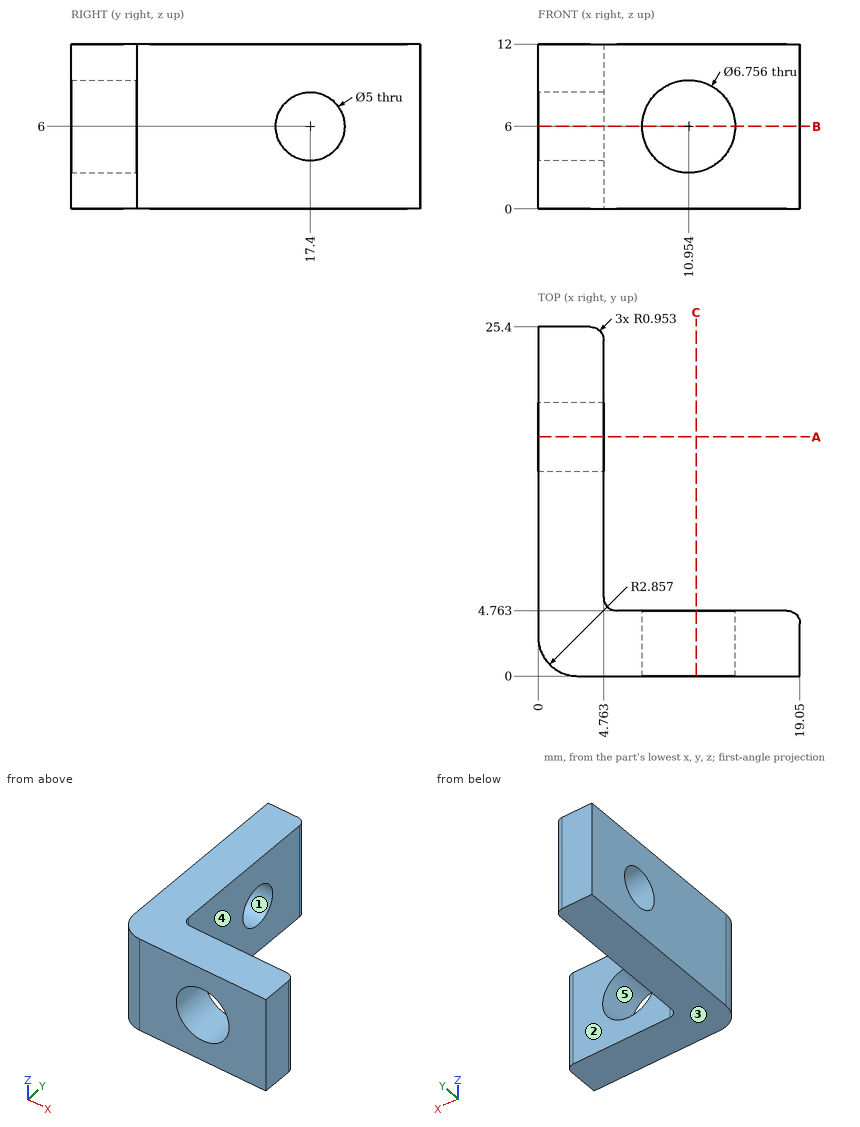
Answer from the drawing. Dimensions are ordinates in mm from the lowest x, y and z of the part. A direction names the side the tool comes from. Round coordinates to 2 decimals unless told otherwise and drop trailing zeros. Write each loop counter-clockwise with the first axis right and the second up, starting at its lowest first coordinate (ties: lowest second). Pieces come first, ordered by that corner, then holes. Notation, with made-up numbers: M -19.5,77 L 36.5,77 A14 cw 36.5,98 Z; hole C 85.5,65 d3. An arc over 180 degrees is marked long. Write each question's results on one line, items separated by ' | '. Start each with the question number.
Item 1: The mould has two halves that part along Z. Classify the marked faces 1, 2 and 3: +Z half, -Z half, draft (parallel to the pull), parting line (faces both ways), or undercut.
Item 2: Find section C-C on x = 11.5. Write down the section's boundary in (y, z).
Item 3: Given pin 1 Ø6 at (x, z) = (10.5, 8) entering from +Y; pin 2 Ø5 at (x, z) = (5, 7) entering from +Y; pin 3 Ø5.5 at (x, z) = (10.95, 6) entering from +Y, each flat-ended and moving along its own axis, determine where each tip first touches the part or whether it passes through.
Item 4: Find section B-B on z = 6. Give the number of separate pieces and of enclosed holes in the cut face, and give its area (3 significant figures).
Item 5: Find section A-A on y = 17.4. Write down the section's boundary in (x, z).
Item 6: Which of the six approach directions +Z, -Z, +X, -X, +Y, -Y give full straight-line access (tool end or side, diameter ignored) to the marked faces 4 and 5?
Item 7: Straight lines are drawn through the part: probe 1 along Z at (x, y) = (1.3, 17.4); probe 2 along X at (y, z) = (20.75, 3); probe 3 along X at (y, z) = (4, 8.75) (1 decimal). For each, find the intervals that lie inside material, in ascending order.
Answer block:
1) face 1: undercut | face 2: draft | face 3: -Z half
2) outline: M 0,0 L 4.76,0 L 4.76,2.67 L 0,2.67 Z; M 0,9.33 L 4.76,9.33 L 4.76,12 L 0,12 Z
3) pin 1: stops at y = 4.76 | pin 2: stops at y = 25.4 | pin 3: passes through
4) separate pieces: 3 | enclosed holes: 0 | area: 131 mm²
5) outline: M 0,0 L 4.76,0 L 4.76,3.5 L 0,3.5 Z; M 0,8.5 L 4.76,8.5 L 4.76,12 L 0,12 Z
6) face 4: +Z, -Z, +X, +Y | face 5: +Y, -Y
7) probe 1: z = 0 to 3.5, 8.5 to 12 | probe 2: x = 0 to 4.76 | probe 3: x = 0 to 9, 12.9 to 19
